Autodesk Inventor part; units mm, degrees
ref_plane "YZ Plane" through (0, 0, 0) normal (1, 0, 0) x (0, 1, 0)
ref_plane "XZ Plane" through (0, 0, 0) normal (0, 1, 0) x (-1, 0, 0)
ref_plane "XY Plane" through (0, 0, 0) normal (0, 0, 1) x (1, 0, 0)
sketch "Sketch1" plane through (0, 0, 0) normal (0, 1, 0) x (-1, 0, 0)
  line L0 (114.3, 114.3) -> (-114.3, 114.3)
  line L1 (-114.3, 114.3) -> (-114.3, -114.3)
  line L2 (-114.3, -114.3) -> (114.3, -114.3)
  line L3 (114.3, -114.3) -> (114.3, 114.3)
  point P0 (0, 0)
  dimension "d0" = 228.6
  dimension "d1" = 228.6
extrude "Extrusion1" add sketch "Sketch1" along normal blind 12.7
sketch "Sketch2" plane through (0, 12.7, 0) normal (0, -1, 0) x (1, 0, 0)
  line L0 (114.3, -114.3) -> (-114.3, -114.3)
  line L1 (-114.3, -114.3) -> (-50.292, -114.3)
  line L2 (-50.292, -114.3) -> (-50.292, -70.358)
  line L3 (-50.292, -70.358) -> (-50.292, -30.353)
  line L4 (-50.292, -30.353) -> (-50.292, 6.731)
  line L5 (-50.292, 6.731) -> (-50.292, 46.736)
  point P0 (0, 0)
  dimension "d4" = 64.008
  dimension "d5" = 43.942
  dimension "d6" = 40.005
  dimension "d7" = 37.084
  dimension "d8" = 40.005
hole "Hole1" at (-50.292, 12.7, 46.736) at (-50.292, 12.7, 6.731) at (-50.292, 12.7, -30.353) at (-50.292, 12.7, -70.358) direction (0, -1, 0) diameter 3.556 depth 25.4 counterbore diameter 6.096 counterbore depth 4.064
sketch "Sketch3" plane through (0, 0, 0) normal (0, -1, 0) x (1, 0, 0)
  line L0 (-114.3, -114.3) -> (-19.304, -114.3)
  line L1 (114.3, -114.3) -> (-114.3, -114.3)
  line L2 (-19.304, -114.3) -> (-19.304, -54.356)
  line L3 (-19.304, -54.356) -> (-19.304, -24.384)
  line L4 (-19.304, -24.384) -> (-19.304, 5.588)
  line L5 (114.3, 114.3) -> (63.5, 114.3)
  line L6 (-114.3, 114.3) -> (114.3, 114.3)
  line L7 (63.5, 114.3) -> (63.5, 74.422)
  line L8 (63.5, 74.422) -> (33.528, 74.422)
  line L9 (63.5, 114.3) -> (63.5, 74.422)
  line L10 (63.5, 74.422) -> (33.528, 74.422)
  line L11 (33.528, 74.422) -> (27.178, 74.422)
  line L12 (27.178, 74.422) -> (-2.794, 74.422)
  point P0 (0, 0)
  dimension "d16" = 94.996
  dimension "d17" = 59.944
  dimension "d18" = 29.972
  dimension "d19" = 29.972
  dimension "d20" = 50.8
  dimension "d21" = 39.878
  dimension "d22" = 29.972
  dimension "d23" = 39.878
  dimension "d24" = 6.35
  dimension "d25" = 29.972
hole "Hole2" at (-2.794, 0, 74.422) at (27.178, 0, 74.422) at (-19.304, 0, 5.588) at (-19.304, 0, -24.384) at (-19.304, 0, -54.356) direction (0, 1, 0) diameter 5.842 depth 25.4
sketch "Sketch4" plane through (0, 12.7, 0) normal (0, 1, 0) x (1, 0, 0)
  line L0 (114.3, -114.3) -> (76.2, -114.3)
  line L1 (-114.3, -114.3) -> (114.3, -114.3)
  line L2 (76.2, -114.3) -> (76.2, -50.292)
  line L3 (76.2, -50.292) -> (36.322, -50.292)
  point P0 (0, 0)
  dimension "d33" = 38.1
  dimension "d34" = 64.008
  dimension "d35" = 39.878
hole "Hole3" at (76.2, 12.7, 50.292) at (36.322, 12.7, 50.292) direction (0, -1, 0) diameter 3.556 depth 25.4 counterbore diameter 6.096 counterbore depth 4.064
sketch "Sketch5" plane through (0, 12.7, 0) normal (0, 1, 0) x (1, 0, 0)
  line L0 (114.3, 114.3) -> (-114.3, 114.3)
  line L1 (-114.3, 114.3) -> (-104.14, 114.3)
  line L2 (-104.14, 114.3) -> (-114.3, 114.3)
  line L3 (-104.14, 114.3) -> (-104.14, 50.8)
  line L4 (-104.14, 50.8) -> (-104.14, -12.7)
  line L5 (-104.14, -12.7) -> (-104.14, -76.2)
  line L6 (-114.3, 114.3) -> (-114.3, 104.14)
  line L7 (-114.3, 114.3) -> (-114.3, -114.3)
  line L8 (-114.3, 104.14) -> (-50.8, 104.14)
  line L9 (-50.8, 104.14) -> (12.7, 104.14)
  line L10 (12.7, 104.14) -> (76.2, 104.14)
  line L11 (-114.3, -114.3) -> (114.3, -114.3)
  line L12 (114.3, -114.3) -> (114.3, -104.14)
  line L13 (114.3, -114.3) -> (114.3, 114.3)
  line L14 (114.3, -104.14) -> (50.8, -104.14)
  line L15 (50.8, -104.14) -> (-12.7, -104.14)
  line L16 (-12.7, -104.14) -> (-76.2, -104.14)
  line L17 (114.3, -114.3) -> (104.14, -114.3)
  line L18 (104.14, -114.3) -> (104.14, -50.8)
  line L19 (104.14, -50.8) -> (104.14, 12.7)
  line L20 (104.14, 12.7) -> (104.14, 76.2)
  point P0 (0, 0)
  dimension "d43" = 10.16
  dimension "d44" = 63.5
  dimension "d45" = 63.5
  dimension "d46" = 63.5
  dimension "d47" = 10.16
  dimension "d48" = 63.5
  dimension "d49" = 90
  dimension "d50" = 63.5
  dimension "d51" = 63.5
  dimension "d52" = 10.16
  dimension "d53" = 63.5
  dimension "d54" = 63.5
  dimension "d55" = 63.5
  dimension "d56" = 10.16
  dimension "d57" = 63.5
  dimension "d58" = 63.5
  dimension "d59" = 63.5
hole "Hole4" [suppressed]
properties part number "sheetmetalbottom"
Geometry check sheet. Reference: the model listing, model coordinates, mm. A direction names the side the tool comes from. Round coordinates to 2 decimals unless told otherwise and drop trailing zeros. Return JSON: item names as keys, results as strings. Group by question number.
Q1. Gauge pin test, flat end, axial feed: pin 1 (5.5 mm diameter, centred on x = -50.292, z = -70.358, fed in from +Y). Record the tip position at first contact, or that the pin passes through.
Q2. Tool access check on faces 4 (the flat face through (2, 6, -114.3)), 5 (the flat face through (78, 8.636, 52)). Record the directions out of +Z, -Z, +X, -X, +Y, -Y that give a thin tool (end or side, any length) a straight path to the whole face; none if there is none.
Q3. Release check for a two-part mould opening along X. For faces 1 (the cylindrical face through (-16.452, 6.439, -53.723)), 2 (the flat face through (114.3, 6, 2)), 3 (the flat face through (2, 0, 2)) record: released by +X, released by -X, zero draft, split by the parting line, or undercut.
Q4. Material ranges on probe 1 along Z at (x, y) = (76.2, 11.55); probe 2 along Z at (x, y) = (77, 0.75); probe 3 along X at (y, z) = (6.75, -53), recorded low to high. Write a range as from..to.
Numbers:
{
 "1": {"pin 1": "y = 8.64"},
 "2": {"face 4": "-Z, +X, -X, +Y, -Y", "face 5": "+Y"},
 "3": {"face 1": "undercut", "face 2": "released by +X", "face 3": "zero draft"},
 "4": {"probe 1": "-114.3..47.24, 53.34..114.3", "probe 2": "-114.3..48.7, 51.88..114.3", "probe 3": "-114.3..-21.89, -16.72..114.3"}
}
